Autodesk Inventor part; units mm, degrees
ref_plane "YZ Plane" through (0, 0, 0) normal (1, 0, 0) x (0, 1, 0)
ref_plane "XZ Plane" through (0, 0, 0) normal (0, 1, 0) x (-1, 0, 0)
ref_plane "XY Plane" through (0, 0, 0) normal (0, 0, 1) x (1, 0, 0)
sketch "Sketch1" plane through (0, 0, 0) normal (1, 0, 0) x (0, 1, 0)
  line L0 (1.27, -4.5) -> (-1.27, -4.5)
  line L1 (-1.27, -4.5) -> (-1.27, 4.5)
  line L2 (-1.27, 4.5) -> (1.27, 4.5)
  line L3 (1.27, 4.5) -> (1.27, -4.5)
  line L4 (1.27, -4.5) -> (-1.27, 4.5) construction
  line L5 (-1.27, -4.5) -> (1.27, 4.5) construction
  point P0 (0, 0)
  point P1 (0, 0)
  dimension "d0" = 9
  dimension "d1" = 2.54
sketch "Sketch2" plane through (0, 0, 0) normal (0, 0, 1) x (1, 0, 0)
  arc A0 (-40.4468, 0) -> (-43.0003, -23.5969) centre (-40.4468, -11.9366) ccw
  arc A1 (36.0209, -40.9014) -> (40.4468, 0) centre (40.4468, -20.6901) ccw
  line L0 (-40.4468, 0) -> (40.4468, 0)
  line L1 (36.0209, -40.9014) -> (-43.0003, -23.5969)
  point P0 (0, 0)
  point P1 (0, 0)
  dimension "d2" = 81.3659
  dimension "d3" = 11.9366
  dimension "d6" = 20.6901
sweep "Sweep1" add profiles "Sketch1" path "Sketch2"
properties part number "53t_Belt" material "Rubber"
CAD build for the part. Positions are in the model's coordinates, mm. A direction names the side the tool comes from. Round coordinates to 2 decimals unless told otherwise and drop trailing zeros. Order: outer loops, then holes, each group sorted by start corner. A loop starts at its lowest first (then second) coordinate and runs counter-clockwise, first axis right, second up.
Item 1: Saw through at A-A on y = -36. Write the cut outline in (x, z), then the cut area to 3 significant figures.
Item 2: Pin check, flat tips, straight feed: pin 1 (4 mm diameter, centred on y = -15, z = 0, fed in from -X); pin 2 (23.5 mm diameter, centred on x = 40.45, y = -20.69, fed in from -Z); pin 3 (1 mm diameter, centred on y = -27, z = 0, fed in from +X); pin 4 (4.5 mm diameter, centred on x = 0, z = 0.5, fed in from -Y). Stop position of each tip, or through.
Item 3: Tool access for faces 4 (the face through (-2.66, -31.13, 0.06)), 5 (the face through (7, -34, -4.5)): list every direction of +Z, -Z, +X, -X, +Y, -Y with a clear straight run to the whole face (end or side of a thin tool).
Item 4: Probe line 1 along X through (y, z) = (-13.5, 2.25); line 2 along Y through (x, z) = (-37, -4); line 3 along X through (y, z) = (-21, -1.75). List the from-to ranges inside material, lowest first.
Item 5: Saw through at C-C on z = -2. Write the cut outline in (x, y).
Item 6: Mould opens along Y. For faces 1 (the face through (-51.073, -11.006, -0.063)), 2 (the face through (-3.21, -33.61, -0.06)), 3 (the face through (-1, 1.27, 0)) say: pulls with the +Y half, pulls with the -Y half, needs draft (parallel to the pull), parting line crosses it, or undercut.
Item 7: Saw through at B-B on x = 45. Write the cut outline in (y, z).
Reported:
1. outline: (7.7, -4.5) - (19.58, -4.5) - (19.58, 4.5) - (7.7, 4.5) - close; (52.39, -4.5) - (56.19, -4.5) - (56.19, 4.5) - (52.39, 4.5) - close
1. area: 141 mm2
2. pin 1: stops at x = -53.61
2. pin 2: passes through
2. pin 3: stops at x = 61.62
2. pin 4: stops at y = -34.81
3. face 4: +Z, -Z
3. face 5: -Z, +X, -X, +Y, -Y
4. line 1: x = -53.56 to -51, 58.49 to 61.2
4. line 2: y = -26.21 to -23.61, -1.27 to 1.27
4. line 3: x = -50.05 to -46.07, 59.86 to 62.4
5. outline: (-43.27, -24.84) - (35.75, -42.14) arc R21.96 ccw (long way) to (40.45, 1.27) - (-40.45, 1.27) arc R13.21 ccw to start; hole (-42.73, -22.36) - (36.29, -39.66) arc R19.42 ccw (long way) to (40.45, -1.27) - (-40.45, -1.27) arc R10.67 ccw to start
6. face 1: undercut
6. face 2: pulls with the -Y half
6. face 3: pulls with the +Y half
7. outline: (-42.17, -4.5) - (-39.57, -4.5) - (-39.57, 4.5) - (-42.17, 4.5) - close; (-1.81, -4.5) - (0.79, -4.5) - (0.79, 4.5) - (-1.81, 4.5) - close
